from build123d import *

# Parameters (mm, degrees)
EXTRUDE_1_DEPTH   = 2
HOLE_WIZARD_M81_D = 9
CHAMFER_1_SIZE    = 2.5


with BuildPart() as part:
    # Эскиз3 → Бобышка-Вытянуть1 (new body)
    with BuildSketch(Plane(origin=(0, 0, 0), x_dir=(1, 0, 0), z_dir=(0, 0, -1))):
        Polygon((0, 0), (112.5, 0), (112.5, 177.355715852), (73.52885683, 199.855715851), (0, 72.5), align=None)
    extrude(amount=EXTRUDE_1_DEPTH)

    # Отверстие с зазором M81 (through all)
    with Locations(Plane(origin=(0, 0, -2), x_dir=(1, 0, 0), z_dir=(0, 0, -1))):
        with Locations((22.5, 22.5), (90, 22.5), (27.5, 75.131397208), (81.764428415, 169.120144266)):
            Hole(HOLE_WIZARD_M81_D / 2)

    # Фаска1
    chamfer_1_edges = [part.edges().sort_by_distance(p)[0] for p in [
        (73.52885683, -199.855715851, -1),
        (112.5, 0, -1),
        (0, 0, -1),
    ]]
    chamfer(chamfer_1_edges, length=CHAMFER_1_SIZE)


solid = part.part
CAD build for the part. Positions are in the model's coordinates, mm. Give positions to 0.01 mm unless a question says otherwise; leave off trailing zeros. Loops run counter-clockwise (first coordinate to the right, second up) from the corner with the lowest first, then second, coordinate; pieces in that order, holes last. Notation, with made-up numbers: M 12.25,19.5 L 63.25,19.5 A12 cw 63.25,32.5 Z; hole C 3,17.5 d4. An arc over 180 degrees is marked long. Answer in a Markdown table with one row per item. Add a question column.
Item 1: Mould opens along X. For faces 1 (the face through (25.081, -78.926, -0.986)), 2 (the face through (55, -79, 0)), 3 (the face through (36.645, -135.972, -0.986)) say: +X half, -X half, draft (parallel to the pull), parting line (faces both ways), or undercut.
Item 2: Band-saw the part on D-D on x = 52. Give the cut face in (y, z).
Item 3: Probe probe 1 along X at (y, z) = (-22.5, -0.5); probe 2 along X at (y, z) = (-25.5, -0.85); probe 3 along Y at (x, z) = (22.5, -0.7). List the from-to ranges inside material, lowest first.
Item 4: Band-saw the part on C-C on z = -1.25. Give the cut face in (x, y), then the cut area to 3 significant figures.
Item 5: Band-saw the part on A-A on y = -22.5. Give the cut face in (x, z).
Item 6: Band-saw the part on B-B on x = 90. Give the cut face in (y, z), then the cut area to 3 significant figures.
Item 7: Drop a flat-ended pin along its axis: P1, Ø8, axis at x = 81.76, y = -169.12, coming from the +Z side. Give the stop position or say it passes through.
Reply:
| question | item | result |
|---|---|---|
| 1 | face 1 | undercut |
| 1 | face 2 | draft |
| 1 | face 3 | -X half |
| 2 | outline | M -162.57,-2 L 0,-2 L 0,0 L -162.57,0 Z |
| 3 | probe 1 | x = 0 to 18, 27 to 85.5, 94.5 to 112.5 |
| 3 | probe 2 | x = 0 to 19.15, 25.85 to 86.65, 93.35 to 112.5 |
| 3 | probe 3 | y = -111.47 to -27, -18 to 0 |
| 4 | outline | M 0,-72.5 L 72.28,-197.69 L 75.69,-198.61 L 112.5,-177.36 L 112.5,-2.5 L 110,0 L 2.5,0 L 0,-2.5 Z; hole C 22.5,-22.5 d9; hole C 27.5,-75.13 d9; hole C 81.76,-169.12 d9; hole C 90,-22.5 d9 |
| 4 | area | 17,100 mm^2 |
| 5 | outline | M 0,-2 L 18,-2 L 18,0 L 0,0 Z; M 27,-2 L 85.5,-2 L 85.5,0 L 27,0 Z; M 94.5,-2 L 112.5,-2 L 112.5,0 L 94.5,0 Z |
| 6 | outline | M -190.35,-2 L -27,-2 L -27,0 L -190.35,0 Z; M -18,-2 L 0,-2 L 0,0 L -18,0 Z |
| 6 | area | 363 mm^2 |
| 7 | P1 | passes through |
